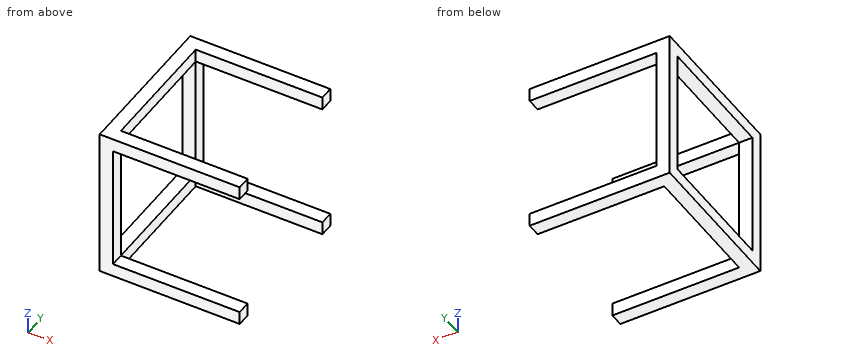
from build123d import *

# Parameters (mm, degrees)
SKETCH_1_W      = 460
SKETCH_1_H      = 460
SKETCH_1_W_2    = 380
SKETCH_1_H_2    = 380
EXTRUDE_2_DEPTH = 40
SKETCH_2_W      = 40
SKETCH_2_H      = 40
EXTRUDE_3_DEPTH = 380


with BuildPart() as part:
    # 草图1 → 凸台-拉伸2 (new body)
    with BuildSketch(Plane(origin=(0, 0, 0), x_dir=(0, 0, -1), z_dir=(1, 0, 0))):
        with Locations((230, 255.532389843)):
            Rectangle(SKETCH_1_W, SKETCH_1_H)
        with Locations((230, 255.532389843)):
            Rectangle(SKETCH_1_W_2, SKETCH_1_H_2, mode=Mode.SUBTRACT)
    extrude(amount=EXTRUDE_2_DEPTH)

    # 草图2 → 凸台-拉伸3 (add)
    with BuildSketch(Plane(origin=(40, 0, 0), x_dir=(0, 0, -1), z_dir=(1, 0, 0))):
        with Locations((20, 465.532389843)):
            Rectangle(SKETCH_2_W, SKETCH_2_H)
        with Locations((440, 465.532389843)):
            Rectangle(SKETCH_2_W, SKETCH_2_H)
        with Locations((440, 45.532389843)):
            Rectangle(SKETCH_2_W, SKETCH_2_H)
        with Locations((20, 45.532389843)):
            Rectangle(SKETCH_2_W, SKETCH_2_H)
    extrude(amount=EXTRUDE_3_DEPTH)


solid = part.part
Input: part model. Units: mm. Frame: model coordinates. Coordinates: 2 decimals unless noted, no trailing zeros. Loops run counter-clockwise (first coordinate to the right, second up) from the corner with the lowest first, then second, coordinate; pieces in that order, holes last.
Q1. Cut plane B-B (x = 88.5). Output: boundary loops of the cut face in (y, z), then the cut area to 3 significant figures.
Q2. Material intervals for line 1 (Z direction, x = 23, y = 74); line 2 (Y direction, x = 391, z = -428), sorted ascending.
Q3. Cut plane A-A (z = -146.5). Output: boundary loops of the cut face in (x, y), then the cut area to 3 significant figures.
Q4. Cut plane D-D (y = 223). Output: boundary loops of the cut face in (x, z), then the cut area to 3 significant figures.
Q5. Cut plane C-C (y = 54). Output: boundary loops of the cut face in (x, z), then the cut area to 3 significant figures.
Q6. Contact query for a flat-ended pin moving along its axis: pin 1 (12 mm diameter, centred on y = 204.5, z = -25, fed in from +X). Output: stop coordinate, or through.
Working result:
1. outline: (25.53, -460) - (65.53, -460) - (65.53, -420) - (25.53, -420) - close; (25.53, -40) - (65.53, -40) - (65.53, 0) - (25.53, 0) - close; (445.53, -460) - (485.53, -460) - (485.53, -420) - (445.53, -420) - close; (445.53, -40) - (485.53, -40) - (485.53, 0) - (445.53, 0) - close
1. area: 6,400 mm2
2. line 1: z = -460 to -420, -40 to 0
2. line 2: y = 25.53 to 65.53, 445.53 to 485.53
3. outline: (0, 25.53) - (40, 25.53) - (40, 65.53) - (0, 65.53) - close; (0, 445.53) - (40, 445.53) - (40, 485.53) - (0, 485.53) - close
3. area: 3,200 mm2
4. outline: (0, -460) - (40, -460) - (40, -420) - (0, -420) - close; (0, -40) - (40, -40) - (40, 0) - (0, 0) - close
4. area: 3,200 mm2
5. outline: (0, -460) - (420, -460) - (420, -420) - (40, -420) - (40, -40) - (420, -40) - (420, 0) - (0, 0) - close
5. area: 48,800 mm2
6. pin 1: stops at x = 40
